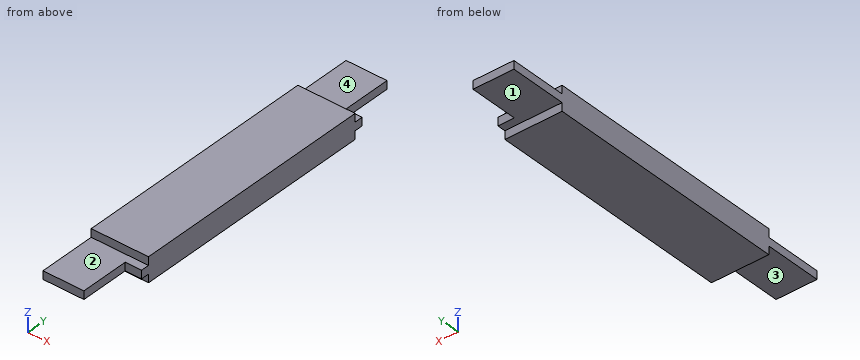
from build123d import *

# Parameters (mm, degrees)
F0_W     = 88.9
F0_H     = 38.1
F1_DEPTH = 190.5
F2_W     = 88.9
F2_H     = 12.7
F3_DEPTH = 12.7
F4_W     = 63.5
F4_H     = 12.7
F5_DEPTH = 76.2


with BuildPart() as f1:
    # F0 (on Front) → F1 (new body)
    with BuildSketch(Plane.XZ):
        with Locations((44.45, 19.05)):
            Rectangle(F0_W, F0_H)
    extrude(amount=F1_DEPTH)

    # F2 (on face) → F3 (join)
    with BuildSketch(Plane.XZ.offset(190.5)):
        with Locations((44.45, 19.05)):
            Rectangle(F2_W, F2_H)
    extrude(amount=F3_DEPTH)

    # F4 (on face) → F5 (join)
    with BuildSketch(Plane.XZ.offset(203.2)):
        with Locations((31.75, 19.05)):
            Rectangle(F4_W, F4_H)
    extrude(amount=F5_DEPTH)

    # F6: F1 across face


with BuildPart() as f1_1:
    add(f1.part)
    add(f1.part.mirror(Plane(origin=(44.45, 0, 19.05), x_dir=(1, 0, 0), z_dir=(0, 1, 0))))


solid = f1_1.part
Can you work these out from the model? Positions are in its coordinate system, mm. Face numbers are marked on the shaded views. A direction names the side the tool comes from. Coordinates: 2 decimals unless noted, no trailing zeros. Write each loop counter-clockwise with the first axis right and the second up, starting at its lowest first coordinate (ties: lowest second). Pieces come first, ordered by that corner, then holes. Notation, with made-up numbers: (28, 14) -> (60, 14) arc R24 ccw to (60, 47) -> close; hole circle Ø4 at (20.25, -39). An arc over 180 degrees is marked (long way). Write item = value, one per line.
(1) Imagine slicing it at C-C (y = -234). Please give me the cut outline in (x, z).
Verdict:
outline = (0, 12.7) -> (63.5, 12.7) -> (63.5, 25.4) -> (0, 25.4) -> close
(2) Imagine slicing it at B-B (z = 17.5). Please give me the cut outline in (x, y), and give its area (3 significant figures).
Verdict:
outline = (0, -279.4) -> (63.5, -279.4) -> (63.5, -203.2) -> (88.9, -203.2) -> (88.9, 203.2) -> (63.5, 203.2) -> (63.5, 279.4) -> (0, 279.4) -> close
area = 45,800 mm^2
(3) Imagine slicing it at A-A (x = 74.5). Please give me the cut outline in (y, z), and give its area (3 significant figures).
Verdict:
outline = (-203.2, 12.7) -> (-190.5, 12.7) -> (-190.5, 0) -> (190.5, 0) -> (190.5, 12.7) -> (203.2, 12.7) -> (203.2, 25.4) -> (190.5, 25.4) -> (190.5, 38.1) -> (-190.5, 38.1) -> (-190.5, 25.4) -> (-203.2, 25.4) -> close
area = 14,800 mm^2
(4) If I drill on probe 1 along Z at (x, y) = (52, -240.5); probe 2 along Y at (x, z) = (58, 26); probe 3 along Y at (x, z) = (66, 19), over which ranges is the centre line in solid material (lowest first)?
Verdict:
probe_1 = 12.7 to 25.4
probe_2 = -190.5 to 190.5
probe_3 = -203.2 to 203.2
(5) Imagine slicing it at D-D (x = 18.5). Please give me the cut outline in (y, z).
Verdict:
outline = (-279.4, 12.7) -> (-190.5, 12.7) -> (-190.5, 0) -> (190.5, 0) -> (190.5, 12.7) -> (279.4, 12.7) -> (279.4, 25.4) -> (190.5, 25.4) -> (190.5, 38.1) -> (-190.5, 38.1) -> (-190.5, 25.4) -> (-279.4, 25.4) -> close
(6) On a 3-axis mill with a long thin cutter (end or side, diameter ignored), from which of +Z, -Z, +X, -X, +Y, -Y can I reach the whole of each face in a straight line? I mean the marked faces 1, 2, 3 and 4. Say none if no direction works.
Verdict:
face_1 = -Z, +X, -X, +Y
face_2 = +Z, +X, -X, -Y
face_3 = -Z, +X, -X, -Y
face_4 = +Z, +X, -X, +Y
(7) For pin 1 (6.5 mm diameter, centred on y = -256.5, z = 20.5, fed in from +X); pin 2 (14 mm diameter, centred on x = 74, z = 16, fed in from +Y); pin 3 (6 mm diameter, centred on x = 41, z = 4, fed in from +Y), each with a flat end and sliding along its axis, tell me the tip position at first contact or that it passes through.
Verdict:
pin_1 = 63.5
pin_2 = 203.2
pin_3 = 190.5
